from build123d import *

# Parameters (mm, degrees)
SKETCH_1_W      = 50
SKETCH_1_H      = 50
SKETCH_1_R      = 14.436913374
SKETCH_1_R_2    = 1.6
EXTRUDE_1_DEPTH = 4
SKETCH_2_W      = 31
SKETCH_2_H      = 50
EXTRUDE_2_DEPTH = 4
SKETCH_3_W      = 50
SKETCH_3_H      = 65
EXTRUDE_3_DEPTH = 4


with BuildPart() as part:
    # 草图1 → 凸台-拉伸1 (new body)
    with BuildSketch(Plane(origin=(0, 0, 0), x_dir=(1, 0, 0), z_dir=(0, 1, 0))):
        Rectangle(SKETCH_1_W, SKETCH_1_H)
        with Locations(Location((0, 0, 0), (0, 0, 270))):
            Circle(SKETCH_1_R, mode=Mode.SUBTRACT)
        with Locations(Location((-17.67766953, -17.67766953, 0), (0, 0, 270))):
            Circle(SKETCH_1_R_2, mode=Mode.SUBTRACT)
        with Locations(Location((17.67766953, -17.67766953, 0), (0, 0, 270))):
            Circle(SKETCH_1_R_2, mode=Mode.SUBTRACT)
        with Locations(Location((17.67766953, 17.67766953, 0), (0, 0, 270))):
            Circle(SKETCH_1_R_2, mode=Mode.SUBTRACT)
        with Locations(Location((-17.67766953, 17.67766953, 0), (0, 0, 270))):
            Circle(SKETCH_1_R_2, mode=Mode.SUBTRACT)
    extrude(amount=EXTRUDE_1_DEPTH)

    # 草图2 → 凸台-拉伸2 (add)
    with BuildSketch(Plane(origin=(0, 0, 0), x_dir=(1, 0, 0), z_dir=(0, 1, 0))):
        with Locations((-40.5, 0)):
            Rectangle(SKETCH_2_W, SKETCH_2_H)
    extrude(amount=EXTRUDE_2_DEPTH)

    # 草图3 → 凸台-拉伸3 (add)
    with BuildSketch(Plane.ZY.offset(55)):
        with Locations((0, 32.5)):
            Rectangle(SKETCH_3_W, SKETCH_3_H)
    extrude(amount=EXTRUDE_3_DEPTH)


solid = part.part
Geometry: final body of the model. Coordinates: model frame, mm. A direction names the side the tool comes from. Give positions to 0.01 mm unless a question says otherwise; leave off trailing zeros. Loops run counter-clockwise (first coordinate to the right, second up) from the corner with the lowest first, then second, coordinate; pieces in that order, holes last. Notation, with made-up numbers: (30, -0.5) - (78, -0.5) arc R25 ccw to (78, 11.5) - close; hole circle Ø8 at (29.25, 21). An arc over 180 degrees is marked (long way). One line per question, with ' | ' between items. Start each with the question number.
(1) Section query A-A on z = 0. Return loops of the section in (x, y), then the cut area to 3 significant figures.
(2) Section query B-B on x = 0. Return loops of the section in (y, z), then the cut area to 3 significant figures.
(3) Ray query, line 1 (X direction, y = 1.2, z = 0); line 2 (X direction, y = 57.5, z = -4); line 3 (Y direction, x = -36, z = -20.5). Return the intervals inside material, ascending. Write a range as from..to.
(4) Pull-direction query (Z, two-part tool) for faces 3 (the cylindrical face through (-16.596, 1.972, 16.498)), 4 (the flat face through (-30, 3, -25)), 5 (the flat face through (-16, 4, 0)); classes: released by +Z, released by -Z, zero draft, split by the parting line, or undercut.
(5) Contact query for flat-ended pins moving along their axis: pin 1 (4 mm diameter, centred on x = -17.68, z = 17.68, fed in from +Y); pin 2 (5 mm diameter, centred on x = -17.68, z = -17.68, fed in from -Y); pin 3 (10 mm diameter, centred on x = -8, y = 12, fed in from -Z); pin 4 (25 mm diameter, centred on y = 45.5, z = -6.5, fed in from +X). Output: stop coordinate, or through.
(6) Reachability of faces 1 (the flat face through (-55, 35, 0)), 2 (the flat face through (25, 2, 0)) from +Z, -Z, +X, -X, +Y, -Y: full face, straight path, thin tool, end or side. Return the list, or none.
(7) Section query C-C on z = 7. Return loops of the section in (x, y).
(8) Section query D-D on x = 12. Return loops of the section in (y, z), then the cut area to 3 significant figures.
The answers:
1) outline: (-59, 0) - (-14.44, 0) - (-14.44, 4) - (-55, 4) - (-55, 65) - (-59, 65) - close; (14.44, 0) - (25, 0) - (25, 4) - (14.44, 4) - close | area: 465 mm2
2) outline: (0, -25) - (4, -25) - (4, -14.44) - (0, -14.44) - close; (0, 14.44) - (4, 14.44) - (4, 25) - (0, 25) - close | area: 84.5 mm2
3) line 1: -59..-14.44, 14.44..25 | line 2: -59..-55 | line 3: 0..4
4) face 3: undercut | face 4: released by -Z | face 5: zero draft
5) pin 1: y = 4 | pin 2: y = 0 | pin 3: through | pin 4: x = -55
6) face 1: +Z, -Z, +X, +Y | face 2: +Z, -Z, +X, +Y, -Y
7) outline: (-59, 0) - (-12.63, 0) - (-12.63, 4) - (-55, 4) - (-55, 65) - (-59, 65) - close; (12.63, 0) - (25, 0) - (25, 4) - (12.63, 4) - close
8) outline: (0, -25) - (4, -25) - (4, -8.03) - (0, -8.03) - close; (0, 8.03) - (4, 8.03) - (4, 25) - (0, 25) - close | area: 136 mm2
